```python
from build123d import *

# Parameters (mm, degrees)
F0_W        = 12.5
F0_H        = 25
F1_DEPTH    = 5.7
F2_W        = 23.5
F2_H        = 2.75
F3_DEPTH    = 25.001
F5_DEPTH    = 13.5
F6_T4_DEPTH = 35.8911325781
F7_R        = 1.65
F8_DEPTH    = 5.701


# Not quite as in the source:
# - a fillet or chamfer that OpenCascade refuses, or shapes differently, is made with other operations: its cross-section is extruded or revolved along the edge and cut away or added


with BuildPart() as f1:
    # F0 (on Top) → F1 (new body)
    with BuildSketch(Plane.XY):
        with Locations((-6.25, 12.5)):
            Rectangle(F0_W, F0_H)
        with Locations((6.25, 12.5)):
            Rectangle(F0_W, F0_H)
    extrude(amount=F1_DEPTH)

    # F2 (on face) → F3 (cut, through all)
    with BuildSketch(Plane.YZ.offset(12.5)):
        with Locations((13.25, 4.325)):
            Rectangle(F2_W, F2_H)
    extrude(amount=-F3_DEPTH, mode=Mode.SUBTRACT)

    # F4 (on face) → F5 (cut)
    with BuildSketch(Plane(origin=(0, 1.5, 0), x_dir=(-1, 0, 0), z_dir=(0, 1, 0))):
        Polygon((9.55, 2.95), (12.5, 0), (12.5, 2.95), align=None)
    extrude(amount=F5_DEPTH, mode=Mode.SUBTRACT)

    # F6: fillet of radius 7 on 1 edges, made by hand


with BuildPart() as f6_tool2:
    # F6_s3 → F6_t4 (new body)
    with BuildSketch(Plane.XZ.offset(-18.695566289)):
        with BuildLine():
            ThreePointArc((-12.5, 0), (-10.0883157712, 4.0898051913), (-5.6217734844, 5.7))
            Line((-5.6217734844, 5.7), (-12.5, 5.7))
            Line((-12.5, 5.7), (-12.5, 0))
        make_face()
    extrude(amount=F6_T4_DEPTH)

    split(bisect_by=Plane.XZ.offset(-15), keep=Keep.TOP)


with BuildPart() as f1_1:
    add(f1.part)

    # F6_t1: cut F6_tool2
    add(f6_tool2.part, mode=Mode.SUBTRACT)

    # F7 (on face) → F8 (cut, through all)
    with BuildSketch(Plane(origin=(0, 0, 0), x_dir=(1, 0, 0), z_dir=(0, 0, -1))):
        with Locations((-1.5, -22)):
            Circle(F7_R)
        with Locations((8.5, -22)):
            Circle(F7_R)
    extrude(amount=-F8_DEPTH, mode=Mode.SUBTRACT)


solid = f1_1.part
```
Geometry: final body of the model. Coordinates: model frame, mm. A direction names the side the tool comes from. Round coordinates to 2 decimals unless told otherwise and drop trailing zeros. Order: outer loops, then holes, each group sorted by start corner. A loop starts at its lowest first (then second) coordinate and runs counter-clockwise, first axis right, second up. Notation, with made-up numbers: (89.25, 45.5) - (116.25, 45.5) arc R9 ccw to (116.25, 53.5) - close; hole circle Ø5 at (88, 49.25). An arc over 180 degrees is marked (long way). Write item = value, one per line. Start each with the question number.
Q1. Pull-direction query (Y, two-part tool) for faces 4 (the flat face through (3, 1, 5.7)), 5 (the flat face through (0, 25, 1)), 6 (the cylindrical face through (8.285, 20.364, 1.454)); classes: +Y half, -Y half, draft (parallel to the pull), parting line (faces both ways), or undercut.
Q2. Ray query, line 1 (X direction, y = 22, z = 0.9); line 2 (Y direction, x = 8.5, z = 0.9); line 3 (Y direction, x = 6.75, z = 3.3). Return the intervals inside material, ascending. Write a range as from..to.
Q3. Cut plane A-A on y = 22. Return the cut outline in (x, z).
Q4. Cut plane D-D on y = 7.25. Return the cut outline in (x, z).
Q5. Pin query (flat end, axial travel): pin 1 (7 mm diameter, centred on x = 5, y = 18, fed in from +Z); pin 2 (1.5 mm diameter, centred on x = 1, z = 4.5, fed in from +Y); pin 3 (2 mm diameter, centred on x = 8.5, y = 22, fed in from +Z). Return the tip coordinate at first contact, or that it passes through.
Q6. Access query for faces 1 (the cylindrical face through (-10.14, 0.761, 4.046)), 2 (the flat face through (-11, 8.2, 1.5)), 3 (the flat face through (0, 13, 2.95)). Directions: +Z, -Z, +X, -X, +Y, -Y. A direction counts if a zero-diameter tool reaches every point of the face in a straight line with its end or side. Return the directions, or none.
Q7. Cut plane C-C on z = 1. Return the cut outline in (x, y), and give its area (3 significant figures).
Q8. Cut plane B-B on x = 8.5. Return the cut outline in (y, z).
Outcome:
q1.face_4 = draft
q1.face_5 = +Y half
q1.face_6 = undercut
q2.line_1 = -12.5..-3.15, 0.15..6.85, 10.15..12.5
q2.line_2 = 0..20.35, 23.65..25
q2.line_3 = 0..1.5
q3.outline = (-12.5, 0) - (-3.15, 0) - (-3.15, 2.95) - (-12.5, 2.95) - close; (0.15, 0) - (6.85, 0) - (6.85, 2.95) - (0.15, 2.95) - close; (10.15, 0) - (12.5, 0) - (12.5, 2.95) - (10.15, 2.95) - close
q4.outline = (-12.5, 0) - (12.5, 0) - (12.5, 2.95) - (-9.55, 2.95) - close
q5.pin_1 = 2.95
q5.pin_2 = 1.5
q5.pin_3 = through
q6.face_1 = +Z, -X, -Y
q6.face_2 = +Z, -X
q6.face_3 = +Z, +X, -X, +Y
q7.outline = (-12.5, 15) - (-11.5, 15) - (-11.5, 1.5) - (-12.23, 1.5) - (-12.23, 0) - (12.5, 0) - (12.5, 25) - (-12.5, 25) - close; hole circle Ø3.3 at (-1.5, 22); hole circle Ø3.3 at (8.5, 22)
q7.area = 594 mm^2
q8.outline = (0, 0) - (20.35, 0) - (20.35, 2.95) - (1.5, 2.95) - (1.5, 5.7) - (0, 5.7) - close; (23.65, 0) - (25, 0) - (25, 2.95) - (23.65, 2.95) - close
